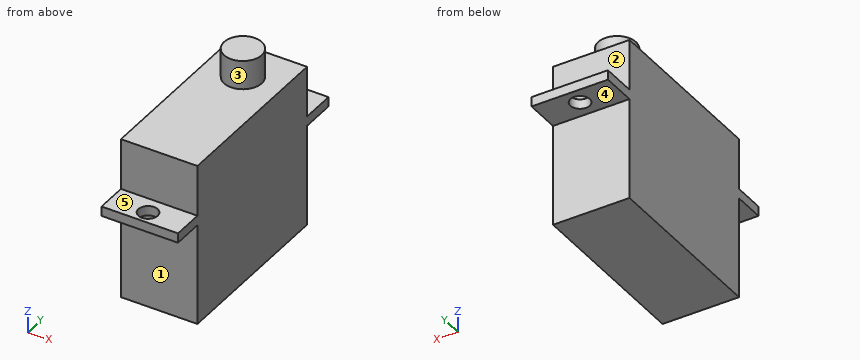
from build123d import *

# Parameters (mm, degrees)
SKETCH1_W           = 16.8
SKETCH1_H           = 18.2
BOSS_EXTRUDE1_DEPTH = 7.91
SKETCH2_W           = 1
SKETCH2_H           = 25
BOSS_EXTRUDE2_DEPTH = 7.91
SKETCH3_R           = 1
CUT_EXTRUDE1_DEPTH  = 21.9
SKETCH4_R           = 1.951580775
BOSS_EXTRUDE3_DEPTH = 3


with BuildPart() as part:
    # Sketch1 → Boss-Extrude1 (new body)
    with BuildSketch(Plane(origin=(0, 0, 0), x_dir=(0, 0, -1), z_dir=(1, 0, 0))):
        with Locations((-6.360008023, 6.524197801)):
            Rectangle(SKETCH1_W, SKETCH1_H)
    extrude(amount=BOSS_EXTRUDE1_DEPTH)

    # Sketch2 → Boss-Extrude2 (add)
    with BuildSketch(Plane(origin=(7.91, 0, 0), x_dir=(0, 0, -1), z_dir=(1, 0, 0))):
        with Locations((-8.970008023, 6.694520813)):
            Rectangle(SKETCH2_W, SKETCH2_H)
    extrude(amount=-BOSS_EXTRUDE2_DEPTH)

    # Sketch3 → Cut-Extrude1 (cut)
    with BuildSketch(Plane.XY.offset(9.470008023)):
        with Locations((3.955, 17.479197801)):
            Circle(SKETCH3_R)
        with Locations((3.955, -4.430802199)):
            Circle(SKETCH3_R)
    extrude(amount=-CUT_EXTRUDE1_DEPTH, mode=Mode.SUBTRACT)

    # Sketch4 → Boss-Extrude3 (add)
    with BuildSketch(Plane.XY.offset(14.760008023)):
        with Locations((3.955, 11.333194866)):
            Circle(SKETCH4_R)
    extrude(amount=BOSS_EXTRUDE3_DEPTH)


solid = part.part
Work out the finished part from the listing and answer in its coordinate system (mm). Face numbers are marked on the shaded views. A direction names the side the tool comes from. Coordinates: 2 decimals unless noted, no trailing zeros. Write each loop counter-clockwise with the first axis right and the second up, starting at its lowest first coordinate (ties: lowest second). Pieces come first, ordered by that corner, then holes.
1. The part is cut by section A-A, the plane x = 3.75. Write down the section's boundary in (y, z).
Results list:
outline: (-5.81, 8.47) - (-5.41, 8.47) - (-5.41, 9.47) - (-5.81, 9.47) - close; (-3.45, 8.47) - (-2.58, 8.47) - (-2.58, -2.04) - (15.62, -2.04) - (15.62, 8.47) - (16.5, 8.47) - (16.5, 9.47) - (15.62, 9.47) - (15.62, 14.76) - (13.27, 14.76) - (13.27, 17.76) - (9.39, 17.76) - (9.39, 14.76) - (-2.58, 14.76) - (-2.58, 9.47) - (-3.45, 9.47) - close; (18.46, 8.47) - (19.19, 8.47) - (19.19, 9.47) - (18.46, 9.47) - close
2. The part is cut by section B-B, the plane x = 1.5. Write down the section's boundary in (y, z).
Results list:
outline: (-5.81, 8.47) - (-2.58, 8.47) - (-2.58, -2.04) - (15.62, -2.04) - (15.62, 8.47) - (19.19, 8.47) - (19.19, 9.47) - (15.62, 9.47) - (15.62, 14.76) - (-2.58, 14.76) - (-2.58, 9.47) - (-5.81, 9.47) - close
3. Consider line 1 along Y through (x, z) = (4.5, 14); line 2 along Z through (x, y) = (6.75, 18); line 3 along Z through (x, y) = (2.5, 4.5). Determine where each line is inside the solid, lowest interval first.
Results list:
line 1: y = -2.58 to 15.62
line 2: z = 8.47 to 9.47
line 3: z = -2.04 to 14.76
4. Flat-ended cylindrical pins translate along their axes: pin 1 (1.5 mm diameter, centred on x = 4, z = 11, fed in from -Y); pin 2 (1.6 mm diameter, centred on x = 5.5, y = -4.5, fed in from -Z); pin 3 (4 mm diameter, centred on x = 4.5, z = 13, fed in from +Y); pin 4 (1.2 mm diameter, centred on x = 3.96, y = -4.43, fed in from +Z). Find the tip coordinate at first contact, or state that the pin passes through.
Results list:
pin 1: stops at y = -2.58
pin 2: stops at z = 8.47
pin 3: stops at y = 15.62
pin 4: passes through
5. The part is cut by section C-C, the plane y = 12.5. Write down the section's boundary in (x, z), and give its area (3 significant figures).
Results list:
outline: (0, -2.04) - (7.91, -2.04) - (7.91, 14.76) - (5.52, 14.76) - (5.52, 17.76) - (2.39, 17.76) - (2.39, 14.76) - (0, 14.76) - close
area: 142 mm2
6. The part is cut by section D-D, the plane z = 6.25. Write down the section's boundary in (x, y), and give its area (3 significant figures).
Results list:
outline: (0, -2.58) - (7.91, -2.58) - (7.91, 15.62) - (0, 15.62) - close
area: 144 mm2
7. For the marked faces 1, 2, 3, 4 and 5, determine the directions among +Z, -Z, +X, -X, +Y, -Y from which every point of the face is accessible in a straight line to the end or side of a thin tool.
Results list:
face 1: -Z, +X, -X, -Y
face 2: +Z, +X, -X, +Y
face 3: +Z
face 4: -Z, +X, -X, +Y
face 5: +Z, +X, -X, -Y
